Geometry check sheet. Reference: drawing and pictorial views, mm from the part's lowest x, y, z. A direction names the side the tool comes from. Round coordinates to 2 decimals unless told otherwise and drop trailing zeros. Order: outer loops, then holes, each group sorted by start corner. A loop starts at its lowest first (then second) coordinate and runs counter-clockwise, first axis right, second up.
Q1. Cross-section at D-D on z = 42. Record the cut outline in (x, y), then the cut area to 3 significant figures.
Q2. Set-up check for the marked faces 1, 2, 3 and 4: record each of +Z, -Z, +X, -X, +Y, -Y from which the full face is reachable in a straight line by a thin tool's end or side.
Q3. Scan lines: probe 1 along Z at (x, y) = (29, 40.5); probe 2 along Z at (x, y) = (27, 25) (1 decimal); probe 3 along Z at (x, y) = (28, 8.5) (1 decimal). Record each from-to range of solid material in increasing order.
Q4. Cross-section at A-A on z = 54.5. Record the cut outline in (x, y), then the cut area to 3 significant figures.
Q5. Cross-section at B-B on y = 36. Record the cut outline in (x, z) (3 decimals), then the cut area to 3 significant figures.
Q6. Depth check by flat-ended pin: P1, Ø4, axis at y = 21, z = 22.5, coming from the +X side; P2, Ø12, axis at x = 39.5, z = 27, coming from the +Y side; P3, Ø4, axis at x = 20, z = 68, coming from the -Y side. Enter the tip coordinate at first touch or a pass-through.
Q7. Mould release check, pull along Z, two halves, no side actions. Record for the marked faces 5, 6 and 7: +Z half, -Z half, draft (parallel to the pull), parting line (faces both ways), or undercut.
Q8. Cross-section at C-C on x = 50. Record the cut outline in (y, z).
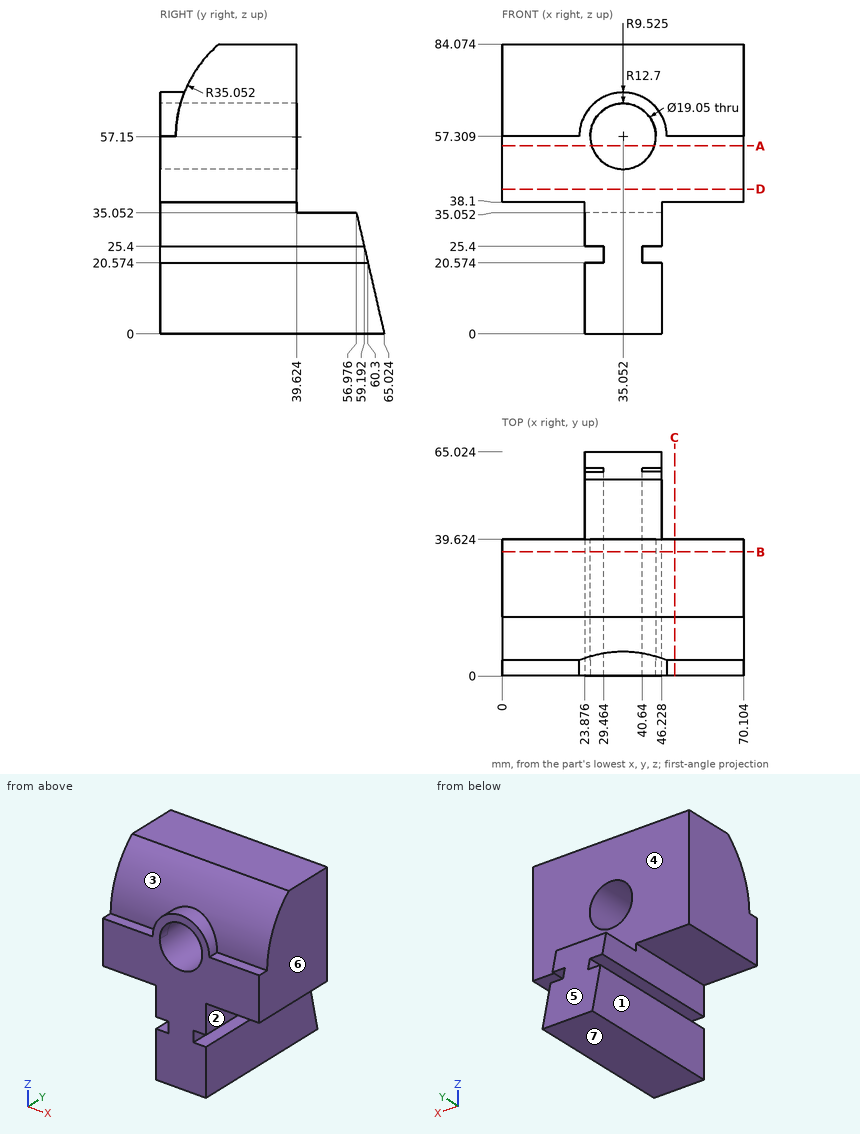
Results found:
1. outline: (0, 0) - (70.1, 0) - (70.1, 39.62) - (0, 39.62) - close
1. area: 2,780 mm2
2. face 1: -Z, -X, +Y, -Y
2. face 2: -Z, +X, +Y, -Y
2. face 3: +Z, -Y
2. face 4: +Z, +X, -X, +Y
3. probe 1: z = 0 to 20.57, 25.4 to 35.05
3. probe 2: z = 0 to 20.6, 25.4 to 52.2, 62.4 to 84.1
3. probe 3: z = 0 to 20.6, 25.4 to 50.9, 63.7 to 73.3
4. outline: (0, 0) - (25.95, 0) - (25.95, 39.62) - (0, 39.62) - close; (44.15, 0) - (70.1, 0) - (70.1, 39.62) - (44.15, 39.62) - close
4. area: 2,060 mm2
5. outline: (0, 38.1) - (23.876, 38.1) - (23.876, 25.4) - (29.464, 25.4) - (29.464, 20.574) - (23.876, 20.574) - (23.876, 0) - (46.228, 0) - (46.228, 20.574) - (40.64, 20.574) - (40.64, 25.4) - (46.228, 25.4) - (46.228, 38.1) - (70.104, 38.1) - (70.104, 84.074) - (0, 84.074) - close; hole circle Ø19.05 at (35.052, 57.309)
5. area: 3,740 mm2
6. P1: stops at x = 46.23
6. P2: stops at y = 60.2
6. P3: stops at y = 5.71
7. face 5: +Z half
7. face 6: draft
7. face 7: -Z half
8. outline: (0, 38.1) - (39.62, 38.1) - (39.62, 84.07) - (17.18, 84.07) arc R35.05 ccw to (4.57, 57.31) - (0, 57.31) - close
